```python
from build123d import *

# Parameters (mm, degrees)
BOSS_EXTRUDE1_DEPTH = 25.654
SKETCH2_W           = 20.6502
SKETCH2_H           = 12.3952
CUT_EXTRUDE1_DEPTH  = 63.010623853
SKETCH3_W           = 42.037
SKETCH3_H           = 20.6502
CUT_EXTRUDE2_DEPTH  = 62.078275718
CUT_EXTRUDE3_DEPTH  = 5.08
SKETCH5_R           = 1.0795
CUT_EXTRUDE4_DEPTH  = 62.078275718
SKETCH6_R           = 1.7145
CUT_EXTRUDE5_DEPTH  = 63.010623853


with BuildPart() as part:
    # Sketch1 → Boss-Extrude1 (new body)
    with BuildSketch(Plane.XY):
        with BuildLine():
            Line((0, 0), (54.0258, 0))
            Line((54.0258, 0), (54.0258, 3.9878))
            Line((54.0258, 3.9878), (51.176616962, 11.038320738))
            ThreePointArc((51.176616962, 11.038320738), (51.065947457, 11.411860999), (51.0286, 11.799656349))
            Line((51.0286, 11.799656349), (51.0286, 15.113))
            Line((51.0286, 15.113), (49.7586, 16.383))
            Line((49.7586, 16.383), (11.2776, 16.383))
            Line((11.2776, 16.383), (10.0076, 15.113))
            Line((10.0076, 15.113), (10.0076, 12.427861529))
            ThreePointArc((10.0076, 12.427861529), (9.790474401, 11.513938717), (9.185498713, 10.795326965))
            Line((9.185498713, 10.795326965), (0, 3.9878))
            Line((0, 3.9878), (0, 0))
        make_face()
    extrude(amount=-BOSS_EXTRUDE1_DEPTH)

    # Sketch2 → Cut-Extrude1 (cut, through all)
    with BuildSketch(Plane(origin=(54.0258, 0, 0), x_dir=(0, 0, -1), z_dir=(1, 0, 0))):
        with Locations((15.3289, 10.1854)):
            Rectangle(SKETCH2_W, SKETCH2_H)
    extrude(amount=-CUT_EXTRUDE1_DEPTH, mode=Mode.SUBTRACT)

    # Sketch3 → Cut-Extrude2 (cut, through all)
    with BuildSketch(Plane(origin=(0, 3.9878, 0), x_dir=(1, 0, 0), z_dir=(0, 1, 0))):
        with Locations((27.0129, 15.3289)):
            Rectangle(SKETCH3_W, SKETCH3_H)
    extrude(amount=-CUT_EXTRUDE2_DEPTH, mode=Mode.SUBTRACT)

    # Sketch4 → Cut-Extrude3 (cut)
    with BuildSketch(Plane.XY):
        with BuildLine():
            Line((6.901956547, 3.937), (10.414, 3.937))
            ThreePointArc((10.414, 3.937), (11.473670222, 4.375929778), (11.9126, 5.4356))
            Line((11.9126, 5.4356), (11.9126, 8.038434234))
            ThreePointArc((11.9126, 8.038434234), (11.088018074, 9.376904105), (9.521699699, 9.242428475))
            Line((9.521699699, 9.242428475), (6.009656246, 6.639594241))
            ThreePointArc((6.009656246, 6.639594241), (5.478912674, 4.965761629), (6.901956547, 3.937))
        make_face()
        with BuildLine():
            Line((47.752, 13.9446), (42.6212, 13.9446))
            ThreePointArc((42.6212, 13.9446), (41.561529778, 13.505670222), (41.1226, 12.446))
            Line((41.1226, 12.446), (41.1226, 5.4356))
            ThreePointArc((41.1226, 5.4356), (41.561529778, 4.375929778), (42.6212, 3.937))
            Line((42.6212, 3.937), (47.752, 3.937))
            ThreePointArc((47.752, 3.937), (48.811670222, 4.375929778), (49.2506, 5.4356))
            Line((49.2506, 5.4356), (49.2506, 12.446))
            ThreePointArc((49.2506, 12.446), (48.811670222, 13.505670222), (47.752, 13.9446))
        make_face()
        with BuildLine():
            Line((13.3096, 12.446), (13.3096, 5.4356))
            ThreePointArc((13.3096, 5.4356), (13.748529778, 4.375929778), (14.8082, 3.937))
            Line((14.8082, 3.937), (19.939, 3.937))
            ThreePointArc((19.939, 3.937), (20.998670222, 4.375929778), (21.4376, 5.4356))
            Line((21.4376, 5.4356), (21.4376, 12.446))
            ThreePointArc((21.4376, 12.446), (20.998670222, 13.505670222), (19.939, 13.9446))
            Line((19.939, 13.9446), (14.8082, 13.9446))
            ThreePointArc((14.8082, 13.9446), (13.748529778, 13.505670222), (13.3096, 12.446))
        make_face()
        with BuildLine():
            Line((22.8346, 12.446), (22.8346, 5.4356))
            ThreePointArc((22.8346, 5.4356), (23.273529778, 4.375929778), (24.3332, 3.937))
            Line((24.3332, 3.937), (38.227, 3.937))
            ThreePointArc((38.227, 3.937), (39.286670222, 4.375929778), (39.7256, 5.4356))
            Line((39.7256, 5.4356), (39.7256, 12.446))
            ThreePointArc((39.7256, 12.446), (39.286670222, 13.505670222), (38.227, 13.9446))
            Line((38.227, 13.9446), (24.3332, 13.9446))
            ThreePointArc((24.3332, 13.9446), (23.273529778, 13.505670222), (22.8346, 12.446))
        make_face()
    extrude(amount=-CUT_EXTRUDE3_DEPTH, mode=Mode.SUBTRACT)

    # Sketch5 → Cut-Extrude4 (cut, through all)
    with BuildSketch(Plane(origin=(0, 3.9878, 0), x_dir=(1, 0, 0), z_dir=(0, 1, 0))):
        with Locations(Location((51.0286, 21.336, 0), (0, 0, 270))):
            Circle(SKETCH5_R)
        with Locations(Location((51.0286, 11.3538, 0), (0, 0, 270))):
            Circle(SKETCH5_R)
        with Locations(Location((2.9972, 11.3538, 0), (0, 0, 90))):
            Circle(SKETCH5_R)
        with Locations(Location((2.9972, 21.336, 0), (0, 0, 90))):
            Circle(SKETCH5_R)
    extrude(amount=-CUT_EXTRUDE4_DEPTH, mode=Mode.SUBTRACT)

    # Sketch6 → Cut-Extrude5 (cut, through all)
    with BuildSketch(Plane.XZ):
        with Locations(Location((45.2501, -2.5019, 0), (0, 0, 270))):
            Circle(SKETCH6_R)
        with Locations(Location((17.2593, -2.5019, 0), (0, 0, 270))):
            Circle(SKETCH6_R)
    extrude(amount=-CUT_EXTRUDE5_DEPTH, mode=Mode.SUBTRACT)


solid = part.part
```
Input: part model. Units: mm. Frame: model coordinates. A direction names the side the tool comes from. Coordinates: 2 decimals unless noted, no trailing zeros. Loops run counter-clockwise (first coordinate to the right, second up) from the corner with the lowest first, then second, coordinate; pieces in that order, holes last.
Q1. Section C-C, the plane y = 2. Return the cut outline in (x, z).
Results are:
outline: (0, -25.65) - (5.99, -25.65) - (5.99, -5) - (48.03, -5) - (48.03, -25.65) - (54.03, -25.65) - (54.03, 0) - (0, 0) - close; hole circle Ø2.16 at (3, -21.34); hole circle Ø2.16 at (3, -11.35); hole circle Ø3.43 at (17.26, -2.5); hole circle Ø3.43 at (45.25, -2.5); hole circle Ø2.16 at (51.03, -21.34); hole circle Ø2.16 at (51.03, -11.35)
Q2. Set-up query: faces 1 (the flat face through (9, 3.937, -2)), 2 (the flat face through (51.029, 13, -2)), 3 (the cylindrical face through (43.729, 15.147, -3.293)), 4 (the flat face through (51, 3.988, -15)), 5 (the flat face through (10.651, 15.757, -2.467)). Return all of +Z, -Z, +X, -X, +Y, -Y with unobstructed straight access to the full face (end or side cutting, diameter ignored); none if empty.
Results are:
face 1: +Z, -Z
face 2: +Z, -Z, +X, +Y
face 3: +Y, -Y
face 4: -Z, +X, -X, +Y
face 5: +Z, -Z, -X, +Y
Q3. Section D-D, the plane z = -2.5. Give the number of separate pieces and of enclosed holes in the cut face, and give its area (3 significant figures).
Results are:
separate pieces: 3
enclosed holes: 2
area: 374 mm2
Q4. Section A-A, the plane x = 33. Return the cut outline in (y, z), and give its area (3 significant figures).
Results are:
outline: (0, -5) - (3.94, -5) - (3.94, 0) - (0, 0) - close; (13.94, -5) - (16.38, -5) - (16.38, 0) - (13.94, 0) - close
area: 31.9 mm2
Q5. Section B-B, the plane z = -19.75. Return the cut outline in (x, y), and give its area (3 significant figures).
Results are:
outline: (0, 0) - (5.99, 0) - (5.99, 3.99) - (0, 3.99) - close; (48.03, 0) - (54.03, 0) - (54.03, 3.99) - (48.03, 3.99) - close
area: 47.8 mm2
Q6. Line query: line 1 along Y through (x, z) = (52, -14.5); line 2 along Z through (x, y) = (20.5, 3.75); line 3 along X through (y, z) = (2.5, -14). Output: solid intervals per line, ascending.
Results are:
line 1: y = 0 to 3.99
line 2: z = -5 to 0
line 3: x = 0 to 5.99, 48.03 to 54.03
Q7. Mould query, pull axis X, two halves, no side actions, for faces 6 (the flat face through (3, 3.988, -15)), 7 (the flat face through (13.31, 9, -2)), 8 (the flat face through (0, 2, -13)). Classes: +X half, -X half, draft (parallel to the pull), parting line (faces both ways), or undercut.
Results are:
face 6: draft
face 7: undercut
face 8: -X half
Q8. Contact query for flat-ended pins moving along their axis: pin 1 (1.3 mm diameter, centred on y = 14, z = -1.5, fed in from -X); pin 2 (6 mm diameter, centred on x = 8.5, y = 11, fed in from -Z); pin 3 (5.5 mm diameter, centred on y = 8, z = -3, fed in from +X). Output: stop coordinate, or through.
Results are:
pin 1: stops at x = 10.01
pin 2: stops at z = -5
pin 3: stops at x = 53.52
